```python
from build123d import *

# Parameters (mm, degrees)
SKETCH1_R           = 1.5
SKETCH1_R_2         = 8.5
BOSS_EXTRUDE1_DEPTH = 2.7
FILLET1_R           = 3
SCALE1_SCALE        = 1.9


with BuildPart() as part:
    # Sketch1 → Boss-Extrude1 (new, symmetric)
    with BuildSketch(Plane.XY):
        with BuildLine():
            Line((10.487675588, 31), (-10.487675588, 31))
            Line((-10.487675588, 31), (-20.108076211, 14.336977332))
            ThreePointArc((-20.108076211, 14.336977332), (-20.407777479, 13.613434467), (-20.51, 12.836977332))
            Line((-20.51, 12.836977332), (-20.51, -12.596152423))
            ThreePointArc((-20.51, -12.596152423), (-20.407777479, -13.372609558), (-20.108076211, -14.096152423))
            Line((-20.108076211, -14.096152423), (-10.348635262, -31))
            Line((-10.348635262, -31), (10.348635262, -31))
            Line((10.348635262, -31), (20.108076211, -14.096152423))
            ThreePointArc((20.108076211, -14.096152423), (20.407777479, -13.372609558), (20.51, -12.596152423))
            Line((20.51, -12.596152423), (20.51, 12.836977332))
            ThreePointArc((20.51, 12.836977332), (20.407777479, 13.613434467), (20.108076211, 14.336977332))
            Line((20.108076211, 14.336977332), (10.487675588, 31))
        make_face()
        with Locations(Location((-6, -27, 0), (0, 0, 180))):
            Circle(SKETCH1_R, mode=Mode.SUBTRACT)
        with Locations(Location((6, -27, 0), (0, 0, 180))):
            Circle(SKETCH1_R, mode=Mode.SUBTRACT)
        with Locations(Location((7.5, -13.4, 0), (0, 0, 180))):
            Circle(SKETCH1_R_2, mode=Mode.SUBTRACT)
        with BuildLine():
            ThreePointArc((-4.5, -13.4), (-8.54, -17.44), (-12.58, -13.4))
            Line((-12.58, -13.4), (-12.58, 1.685368783))
            ThreePointArc((-12.58, 1.685368783), (-10.18215631, 2.859423407), (-8.730303993, 5.1))
            Line((-8.730303993, 5.1), (8.729875369, 5.1))
            ThreePointArc((8.729875369, 5.1), (10.179804764, 2.860963681), (12.574584064, 1.685969643))
            ThreePointArc((12.574584064, 1.685969643), (14.121431526, -0.726790857), (11.622623122, -2.13039581))
            ThreePointArc((11.622623122, -2.13039581), (11.545720037, -2.104624526), (11.469942926, -2.075709596))
            ThreePointArc((11.469942926, -2.075709596), (0.558793877, -3.611248417), (-4.5, -13.4))
        make_face(mode=Mode.SUBTRACT)
        with Locations(Location((-13.5, 6.6, 0), (0, 0, 180))):
            Circle(SKETCH1_R, mode=Mode.SUBTRACT)
        with BuildLine():
            Line((8.729875369, 8.1), (-8.730303993, 8.1))
            ThreePointArc((-8.730303993, 8.1), (-10.179901517, 10.338575405), (-12.574074074, 11.513518208))
            ThreePointArc((-12.574074074, 11.513518208), (-0.00020804, 20.099999998), (12.57392263, 11.513905748))
            ThreePointArc((12.57392263, 11.513905748), (10.179553129, 10.338812856), (8.729875369, 8.1))
        make_face(mode=Mode.SUBTRACT)
        with Locations(Location((-5.24, 27, 0), (0, 0, 180))):
            Circle(SKETCH1_R, mode=Mode.SUBTRACT)
        with Locations(Location((13.5, 6.6, 0), (0, 0, 180))):
            Circle(SKETCH1_R, mode=Mode.SUBTRACT)
        with Locations(Location((5.24, 27, 0), (0, 0, 180))):
            Circle(SKETCH1_R, mode=Mode.SUBTRACT)
    extrude(amount=BOSS_EXTRUDE1_DEPTH, both=True)

    # Fillet1
    fillet1_edges = [part.edges().sort_by_distance(p)[0] for p in [
        (-10.487675588, 31, 0),
        (10.487675588, 31, 0),
        (10.348635262, -31, 0),
        (-10.348635262, -31, 0),
    ]]
    fillet(fillet1_edges, radius=FILLET1_R)


with BuildPart() as part_1:
    # Scale1: scaled about (-0.489793852, 0.73928426, 0)
    add(part.part.scale(SCALE1_SCALE).moved(Location((0.440814467, -0.665355834, 0))))


solid = part_1.part
```
Check sheet for the modelled part. Datum: model origin and axes. Units: mm. A direction names the side the tool comes from. Give positions to 0.01 mm unless a question says otherwise; leave off trailing zeros. Write each loop counter-clockwise with the first axis right and the second up, starting at its lowest first coordinate (ties: lowest second). Pieces come first, ordered by that corner, then holes.
Item 1: Scan lines: L1, parallel to X at y = -19.5, z = 2; L2, parallel to Y at x = -11, z = -1.75; L3, parallel to Y at x = 9.5, z = -1.5. Record each from-to range of solid material in increasing order.
Item 2: Cross-section at C-C (y = 16.5). Enter the section's corners in (x, z), and give its area (3 significant figures).
Item 3: Access from +Z, -Z, +X, -X, +Y, -Y to the whole of each face (thin tool, end or side, straight path). Record for faces 1 (the face through (1, 14.725, 0)), 2 (the face through (0, 13, 5.13)).
Item 4: Cross-section at A-A (y = -32). Enter the section's corners in (x, z).
Item 5: Cross-section at B-B (x = 3). Enter the section's corners in (y, z).
Item 6: Gauge pin test, flat ends, axial feed: pin 1 (9 mm diameter, centred on x = 10.4, y = 50.63, fed in from +Z); pin 2 (6 mm diameter, centred on y = -41, z = 3, fed in from -X); pin 3 (4 mm diameter, centred on x = -18.5, z = 4, fed in from -Y). Record the tip position at first contact, or that the pin passes through.
Item 7: Draft check along Y on faces 3 (the face through (0, -59.565, 0)), 4 (the face through (0, 13, -5.13)), 5 (the face through (-19.01, 57.49, 0.07)), 6 (the face through (1.752, -7.352, 0.072)). Enter one of: released by +Y, released by -Y, zero draft, split by the parting line, or undercut.
Item 8: Cross-section at D-D (z = 2). Count the separate pieces of the cut face and the enclosed holes in it, and give its area (3 significant figures).
Report:
1. L1: x = -38.53 to -23.46, -7.13 to -0.04, 29.42 to 39.41
1. L2: y = -59.57 to -54.82, -49.12 to -32.13, 9.02 to 14.72, 34.83 to 48.2, 53.07 to 58.23
1. L3: y = -59.57 to -53.59, -50.34 to -41.42, -10.83 to -3.92, 9.02 to 14.72, 35.87 to 47.93, 53.34 to 58.23
2. outline: (-38.53, -5.13) - (-16.91, -5.13) - (-16.91, 5.13) - (-38.53, 5.13) - close; (17.79, -5.13) - (39.41, -5.13) - (39.41, 5.13) - (17.79, 5.13) - close
2. area: 444 mm2
3. face 1: +Z, -Z
3. face 2: +Z, +X, -X, +Y, -Y
4. outline: (-35.14, -5.13) - (-20.73, -5.13) - (-20.73, 5.13) - (-35.14, 5.13) - close; (-10.84, -5.13) - (-0.35, -5.13) - (-0.35, 5.13) - (-10.84, 5.13) - close; (29.73, -5.13) - (36.02, -5.13) - (36.02, 5.13) - (29.73, 5.13) - close
5. outline: (-59.57, -5.13) - (-37.27, -5.13) - (-37.27, 5.13) - (-59.57, 5.13) - close; (-14.98, -5.13) - (-6.55, -5.13) - (-6.55, 5.13) - (-14.98, 5.13) - close; (9.02, -5.13) - (14.72, -5.13) - (14.72, 5.13) - (9.02, 5.13) - close; (37.4, -5.13) - (58.23, -5.13) - (58.23, 5.13) - (37.4, 5.13) - close
6. pin 1: stops at z = 5.13
6. pin 2: stops at x = -31.67
6. pin 3: stops at y = -59.54
7. face 3: released by -Y
7. face 4: zero draft
7. face 5: released by +Y
7. face 6: undercut
8. separate pieces: 1
8. enclosed holes: 9
8. area: 5,010 mm2
